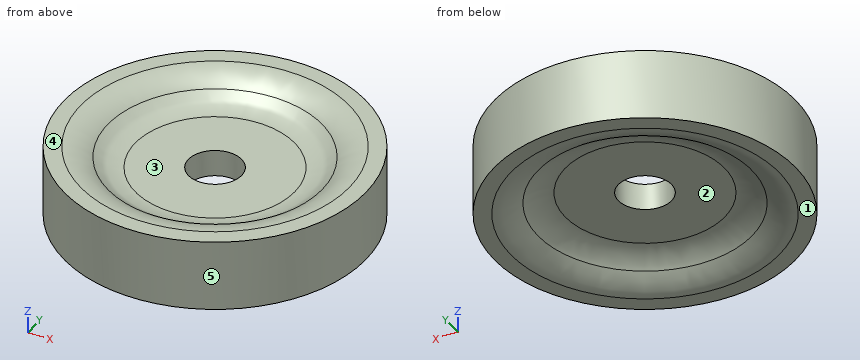
```python
from build123d import *


with BuildPart() as part:
    # Croquis2 → Revolución1 (revolve)
    with BuildSketch(Plane(origin=(0, 0, 0), x_dir=(1, 0, 0), z_dir=(0, 1, 0))):
        with BuildLine():
            Line((15, -7.5), (15, 7.5))
            Line((15, 7.5), (45, 7.5))
            ThreePointArc((45, 7.5), (53.291561976, 9.122316128), (60.360257159, 13.75))
            ThreePointArc((60.360257159, 13.75), (67.428952343, 18.377683872), (75.720514319, 20))
            Line((75.720514319, 20), (85, 20))
            Line((85, 20), (85, -20))
            Line((85, -20), (75.720514319, -20))
            ThreePointArc((75.720514319, -20), (67.428952343, -18.377683872), (60.360257159, -13.75))
            ThreePointArc((60.360257159, -13.75), (53.291561976, -9.122316128), (45, -7.5))
            Line((45, -7.5), (15, -7.5))
        make_face()
    revolve(axis=Axis((0, 0, 0), (0, 0, -1)))


solid = part.part
```
Input: part model. Units: mm. Frame: model coordinates. Face numbers are marked on the shaded views. A direction names the side the tool comes from. Give positions to 0.01 mm unless a question says otherwise; leave off trailing zeros. Loops run counter-clockwise (first coordinate to the right, second up) from the corner with the lowest first, then second, coordinate; pieces in that order, holes last.
1) Section query D-D on z = -10.5. Return the cut outline in (x, y), and give its area (3 significant figures).
A:
outline: circle Ø170 at (0, 0); hole circle Ø112.18 at (0, 0)
area: 12,800 mm2
2) Reachability of the marked faces 1 and 2 from +Z, -Z, +X, -X, +Y, -Y: full face, straight path, thin tool, end or side. Return the list, or none.
A:
face 1: -Z, +X, -X, +Y, -Y
face 2: -Z
3) Contact query for flat-ended pins moving along their axis: pin 1 (1.5 mm diameter, centred on y = -23, z = 5.5, fed in from -X); pin 2 (1.5 mm diameter, centred on y = -55.5, z = -5, fed in from +X); pin 3 (10 mm diameter, centred on x = -67.5, y = -3, fed in from -Z). Output: stop coordinate, or through.
A:
pin 1: stops at x = -82.04
pin 2: stops at x = 65.02
pin 3: stops at z = -19.77
4) Line query: L1, parallel to X at y = 0, z = 3.25; L2, parallel to X at y = -10, z = -11. Output: solid intervals per line, ascending.
A:
L1: x = -85 to -15, 15 to 85
L2: x = -84.41 to -56.02, 56.02 to 84.41
5) Mould query, pull axis Y, two halves, no side actions, for the marked faces 3, 4 and 5. Classes: released by +Y, released by -Y, zero draft, split by the parting line, or undercut.
A:
face 3: undercut
face 4: zero draft
face 5: split by the parting line
6) Section query A-A on y = 0. Return the cut outline in (x, z), and give its area (3 significant figures).
A:
outline: (-85, -20) - (-75.72, -20) arc R22 ccw to (-60.36, -13.75) arc R22 cw to (-45, -7.5) - (-15, -7.5) - (-15, 7.5) - (-45, 7.5) arc R22 cw to (-60.36, 13.75) arc R22 ccw to (-75.72, 20) - (-85, 20) - close; (15, -7.5) - (45, -7.5) arc R22 cw to (60.36, -13.75) arc R22 ccw to (75.72, -20) - (85, -20) - (85, 20) - (75.72, 20) arc R22 ccw to (60.36, 13.75) arc R22 cw to (45, 7.5) - (15, 7.5) - close
area: 3,330 mm2
7) Section query C-C on z = 4.5. Return the cut outline in (x, y), and give its area (3 significant figures).
A:
outline: circle Ø170 at (0, 0); hole circle Ø30 at (0, 0)
area: 22,000 mm2
